Read the model definition and answer for the solid it produces. Units are mm, in the model's axes. Coordinates: 2 decimals unless noted, no trailing zeros. Write each loop counter-clockwise with the first axis right and the second up, starting at its lowest first coordinate (ties: lowest second). Pieces come first, ordered by that corner, then holes. Notation, with made-up numbers: (-5.5, 4.5) - (3.5, 4.5) arc R16 ccw to (3.5, 22.5) - close; hole circle Ø3 at (-14, 20.25). An arc over 180 degrees is marked (long way). Return JSON: item names as keys, results as strings.
```python
from build123d import *

# Parameters (mm, degrees)
SKETCH_1_W          = 30
SKETCH_1_H          = 3
EXTRUDE_1_DEPTH     = 3
SKETCH_2_R          = 1.75
CUT_EXTRUDE_1_DEPTH = 10


with BuildPart() as part:
    # Эскиз1 → Бобышка-Вытянуть1 (new body)
    with BuildSketch(Plane.XY):
        Polygon((-27.5, 50), (-27.5, -50), (27.5, -50), (27.5, 50), (15, 50), (15, 47), (-15, 47), (-15, 50), align=None)
        with Locations((0, 48.5)):
            Rectangle(SKETCH_1_W, SKETCH_1_H)
        with Locations((0, 51.5)):
            Rectangle(SKETCH_1_W, SKETCH_1_H)
    extrude(amount=EXTRUDE_1_DEPTH)

    # Эскиз2 → Вырез-Вытянуть1 (cut)
    with BuildSketch(Plane.XY.offset(3)):
        with Locations((-8, 8)):
            Circle(SKETCH_2_R)
        with Locations((-8, -8)):
            Circle(SKETCH_2_R)
    extrude(amount=-CUT_EXTRUDE_1_DEPTH, mode=Mode.SUBTRACT)


solid = part.part
```
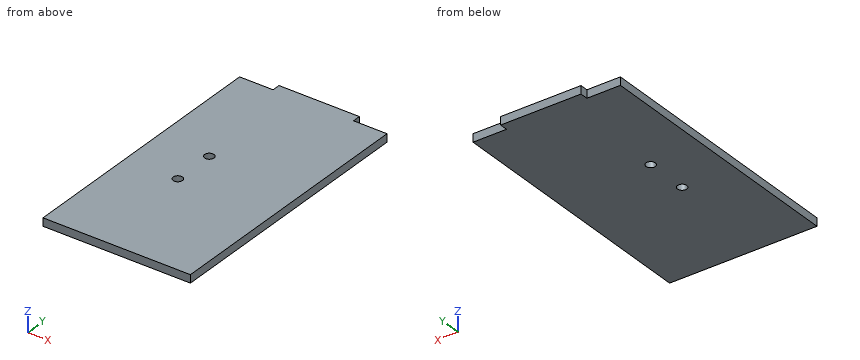
(1) Straight lines are drawn through the part: line 1 (Y direction, x = -8, z = 1.9); line 2 (Y direction, x = 20, z = 2.5); line 3 (Y direction, x = -9, z = 1.95). For each, find the intervals that lie inside material, in ascending order. Write a range as from..to.
Answer:
{"line 1": "-50..-9.75, -6.25..6.25, 9.75..53", "line 2": "-50..50", "line 3": "-50..-9.44, -6.56..6.56, 9.44..53"}
(2) Flat-ended cylindrical pins translate along their axes: P1, Ø0.9, axis at y = 51.5, z = 2, coming from the -X side; P2, Ø0.9, axis at x = 22.5, z = 1, coming from the +Y side; P3, Ø5.5, axis at x = -8, y = 8, coming from the +Z side. Find the tip coordinate at first contact, or state that the pin passes through.
Answer:
{"P1": "x = -15", "P2": "y = 50", "P3": "z = 3"}
(3) A cutting plane is placed at D-D (x = 22). Determine the outline of the cut face in (y, z), and give its area (3 significant figures).
Answer:
{"outline": "(-50, 0) - (50, 0) - (50, 3) - (-50, 3) - close", "area": "300 mm²"}
(4) A cutting plane is placed at C-C (x = -7.5). Determine the outline of the cut face in (y, z).
Answer:
{"outline": "(-50, 0) - (-9.68, 0) - (-9.68, 3) - (-50, 3) - close; (-6.32, 0) - (6.32, 0) - (6.32, 3) - (-6.32, 3) - close; (9.68, 0) - (53, 0) - (53, 3) - (9.68, 3) - close"}
(5) A cutting plane is placed at A-A (y = -8). Determine the outline of the cut face in (x, z).
Answer:
{"outline": "(-27.5, 0) - (-9.75, 0) - (-9.75, 3) - (-27.5, 3) - close; (-6.25, 0) - (27.5, 0) - (27.5, 3) - (-6.25, 3) - close"}
(6) A cutting plane is placed at B-B (z = 1.6). Determine the outline of the cut face in (x, y).
Answer:
{"outline": "(-27.5, -50) - (27.5, -50) - (27.5, 50) - (15, 50) - (15, 53) - (-15, 53) - (-15, 50) - (-27.5, 50) - close; hole circle Ø3.5 at (-8, -8); hole circle Ø3.5 at (-8, 8)"}
